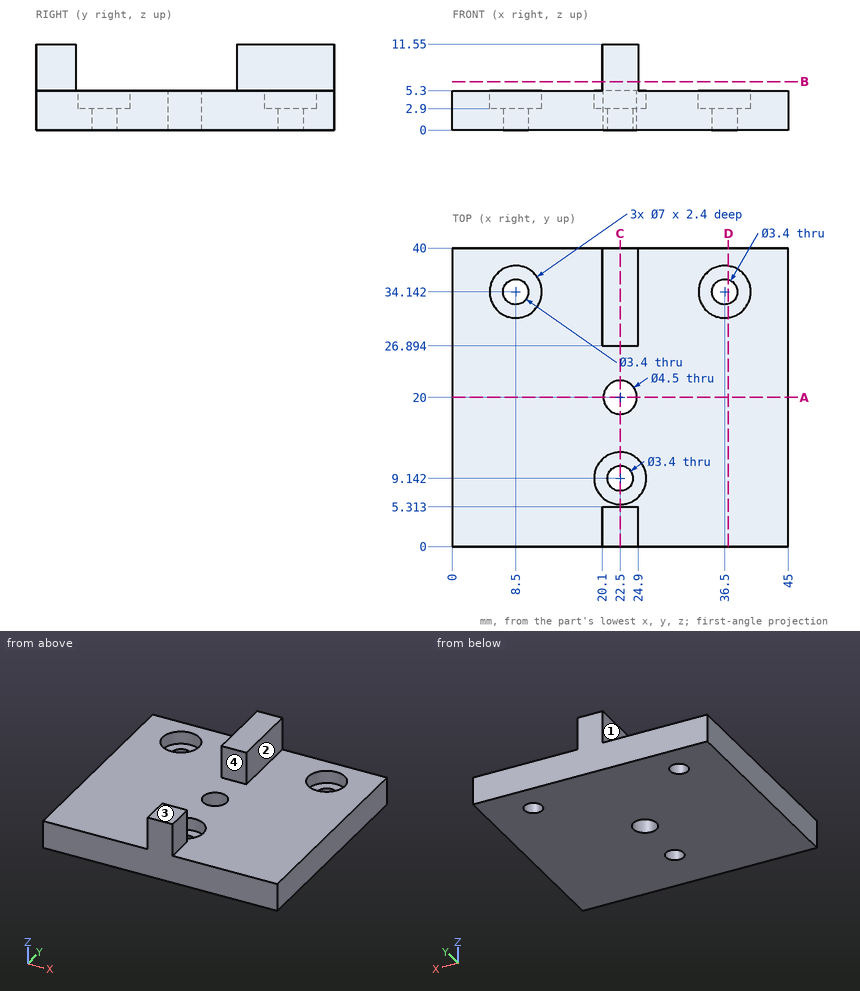
Design review of the part shown in the three views and the two pictorial views. Dimensions are in mm from the part's minimum x, y and z. A direction names the side the tool comes from. Coordinates: 2 decimals unless noted, no trailing zeros. Loops run counter-clockwise (first coordinate to the right, second up) from the corner with the lowest first, then second, coordinate; pieces in that order, holes last. Notation, with made-up numbers: (53.25, 25) -> (83.25, 25) arc R16 cw to (83.25, 51) -> close; hole circle Ø5 at (-10.5, -7). An arc over 180 degrees is marked (long way). Answer as CSV lines item,"result".
Item 1: Insertion check: pin 1 (6.5 mm diameter, centred on x = 22.5, y = 9.14, fed in from +Z); pin 2 (2 mm diameter, centred on x = 36.5, y = 34.14, fed in from +Z); pin 3 (2 mm diameter, centred on y = 30.5, z = 6.5, fed in from -X); pin 4 (5 mm diameter, centred on x = 35, y = 28.5, fed in from +Z). Each pin has a flat end and moves straight along its axis. Give the tip position at first contact, or say it passes through.
Results below:
pin 1,"stops at z = 2.9"
pin 2,"passes through"
pin 3,"stops at x = 20.1"
pin 4,"stops at z = 5.3"
Item 2: Take a section at A-A, the plane y = 20. State the section outline as (x, z) points, and give its area (3 significant figures).
Results below:
outline,"(0, 0) -> (20.25, 0) -> (20.25, 5.3) -> (0, 5.3) -> close; (24.75, 0) -> (45, 0) -> (45, 5.3) -> (24.75, 5.3) -> close"
area,"215 mm2"
Item 3: For L1, parallel to Y at x = 22.5, z = 4.85; L2, parallel to Y at x = 22.5, z = 0.75; L3, parallel to Y at x = 36.5, z = 1.8, list the stretches that pass through material, from the lowest coordinate up.
Results below:
L1,"y = 0 to 5.64, 12.64 to 17.75, 22.25 to 40"
L2,"y = 0 to 7.44, 10.84 to 17.75, 22.25 to 40"
L3,"y = 0 to 32.44, 35.84 to 40"
Item 4: Take a section at D-D, the plane x = 37. State the section outline as (y, z) points, and give its area (3 significant figures).
Results below:
outline,"(0, 0) -> (32.52, 0) -> (32.52, 2.9) -> (30.68, 2.9) -> (30.68, 5.3) -> (0, 5.3) -> close; (35.77, 0) -> (40, 0) -> (40, 5.3) -> (37.61, 5.3) -> (37.61, 2.9) -> (35.77, 2.9) -> close"
area,"186 mm2"
Item 5: Machinability: for the marked faces 1, 2, 3 and 4, which of the approach directions +Z, -Z, +X, -X, +Y, -Y give a long, thin tool a straight path to every point of the face, cutting with its end or side? Answer none if there is none.
Results below:
face 1,"+Z, -X, +Y, -Y"
face 2,"+Z, +X, +Y, -Y"
face 3,"+Z, +X, -X, +Y, -Y"
face 4,"+Z, +X, -X"
Item 6: Take a section at B-B, the plane z = 6.5. State the section outline as (x, y) points, and give its area (3 significant figures).
Results below:
outline,"(20.1, 0) -> (24.9, 0) -> (24.9, 5.31) -> (20.1, 5.31) -> close; (20.1, 26.89) -> (24.9, 26.89) -> (24.9, 40) -> (20.1, 40) -> close"
area,"88.4 mm2"
Item 7: Take a section at C-C, the plane x = 22.5. State the section outline as (y, z) points.
Results below:
outline,"(0, 0) -> (7.44, 0) -> (7.44, 2.9) -> (5.64, 2.9) -> (5.64, 5.3) -> (5.31, 5.3) -> (5.31, 11.55) -> (0, 11.55) -> close; (10.84, 0) -> (17.75, 0) -> (17.75, 5.3) -> (12.64, 5.3) -> (12.64, 2.9) -> (10.84, 2.9) -> close; (22.25, 0) -> (40, 0) -> (40, 11.55) -> (26.89, 11.55) -> (26.89, 5.3) -> (22.25, 5.3) -> close"
